```python
from build123d import *

# Parameters (mm, degrees)
F1_DEPTH = 38.1
F2_R     = 36.5125
F2_R_2   = 31.75
F3_DEPTH = 50.8
F5_DEPTH = 127


with BuildPart() as f1:
    # F0 (on Right) → F1 (new body)
    with BuildSketch(Plane.YZ):
        with BuildLine():
            Line((50.8, 0), (0, 0))
            Line((0, 0), (0, -3.175))
            Line((0, -3.175), (-127, -3.175))
            Line((-127, -3.175), (-127, 66.675))
            Line((-127, 66.675), (0, 66.675))
            Line((0, 66.675), (0, 63.5))
            Line((0, 63.5), (50.8, 63.5))
            Line((50.8, 63.5), (50.8, 76.2))
            Line((50.8, 76.2), (-127, 109.855))
            ThreePointArc((-127, 109.855), (-164.16102, 31.75), (-127, -46.355))
            Line((-127, -46.355), (50.8, -12.7))
            Line((50.8, -12.7), (50.8, 0))
        make_face()
    extrude(amount=F1_DEPTH)

    # F2 (on face) → F3 (join)
    with BuildSketch(Plane(origin=(0, 50.8, 0), x_dir=(-1, 0, 0), z_dir=(0, 1, 0))):
        with Locations((-19.05, 31.75)):
            Circle(F2_R)
        with Locations((-19.05, 31.75)):
            Circle(F2_R_2, mode=Mode.SUBTRACT)
    extrude(amount=-F3_DEPTH)

    # F4 (on face) → F5 (cut)
    with BuildSketch(Plane.YZ.offset(38.1)):
        with BuildLine():
            Line((-153.815218, 76.2), (50.8, 76.2))
            Line((50.8, 76.2), (-127, 109.855))
            ThreePointArc((-127, 109.855), (-142.227029, 94.477155), (-153.815218, 76.2))
        make_face()
    extrude(amount=-F5_DEPTH, mode=Mode.SUBTRACT)


solid = f1.part
```
Could you check a few things on this model? Use its own coordinates, in mm. A direction names the side the tool comes from. Round coordinates to 2 decimals unless told otherwise and drop trailing zeros. Order: outer loops, then holes, each group sorted by start corner. A loop starts at its lowest first (then second) coordinate and runs counter-clockwise, first axis right, second up. Notation, with made-up numbers: M 3,83.25 L 37,83.25 A23 cw 37,109.25 Z; hole C -1,-32 d2. An arc over 180 degrees is marked long. One line per question, with ' | ' between items. Start each with the question number.
(1) Suppose I cut it at D-D on x = 19.05. List the corners of the cut face in (y, z) for me (3 decimals).
(2) For faces 1 (the face through (27.3, 0, 0.9)), 2 (the face through (19, -53, 76.2)), which set-ups out of +Z, -Z, +X, -X, +Y, -Y let a thin tool reach every point of the face, with its end or its side?
(3) Suppose I cut it at A-A on z = 31.75. List the corners of the cut face in (x, y) for me.
(4) For P1, Ø2, axis at y = 23.5, z = 53, coming from the +X side; P2, Ø21, axis at x = 28.5, z = 46, coming from the -Y side; P3, Ø10, axis at x = 28, y = -100.5, coming from the -Z side, each with a flat end and sliding along its axis, tell me the tip position at first contact or that it passes through.
(5) Please list where these lines run through material, in increasing order: line 1 along X through (y, z) = (21.5, 31.75); line 2 along X through (y, z) = (-57, -12.5); line 3 along Y through (x, z) = (-3, 56).
(6) Suppose I cut it at B-B on y = -90. List the corners of the cut face in (x, z) for me (3 decimals), then the cut area to 3 significant figures.
(7) Thinking about a two-plate mould opening in Y: for faces 3 (the face through (19, -63, -3.175)), 4 (the face through (4.4, 25.76, 3.58)), 5 (the face through (18.783, -39.345, -29.763)), which applies, +Y half, -Y half, draft (parallel to the pull), parting line (faces both ways), or undercut?
(8) Suppose I cut it at C-C on x = -2.5. List the corners of the cut face in (y, z) for me.
Geometry results:
1) outline: M -153.815,76.2 A100.661 ccw -127,-46.355 L 50.8,-12.7 L 50.8,0 L 0,0 L 0,-3.175 L -127,-3.175 L -127,66.675 L 0,66.675 L 0,63.5 L 50.8,63.5 L 50.8,76.2 Z
2) face 1: +X, -X | face 2: +Z, +X, -X, +Y, -Y
3) outline: M -17.46,0 L -12.7,0 L -12.7,50.8 L -17.46,50.8 Z; M 0,-164.16 L 38.1,-164.16 L 38.1,-127 L 0,-127 Z; M 50.8,0 L 55.56,0 L 55.56,50.8 L 50.8,50.8 Z
4) P1: x = 49.43 | P2: y = -164.09 | P3: z = -42.29
5) line 1: -17.46 to -12.7, 50.8 to 55.56 | line 2: 0 to 38.1 | line 3: 0 to 50.8
6) outline: M 0,-39.351 L 38.1,-39.351 L 38.1,-3.175 L 0,-3.175 Z; M 0,66.675 L 38.1,66.675 L 38.1,76.2 L 0,76.2 Z | area: 1,740 mm²
7) face 3: undercut | face 4: draft | face 5: +Y half
8) outline: M 0,2.28 L 50.8,2.28 L 50.8,8.43 L 0,8.43 Z; M 0,55.07 L 50.8,55.07 L 50.8,61.22 L 0,61.22 Z
